```python
from build123d import *

# Parameters (mm, degrees)
ESQUISSE1_W             = 20
ESQUISSE1_H             = 20
BOSS_EXTRU_1_DEPTH      = 4
ESQUISSE4_W             = 20
ESQUISSE4_H             = 20
ESQUISSE4_W_2           = 12
ESQUISSE4_H_2           = 12
BOSS_EXTRU_2_DEPTH      = 16
ENL_V_MAT_EXTRU_2_DEPTH = 25
ENL_V_MAT_EXTRU_3_DEPTH = 25
CHANFREIN1_SIZE         = 2


with BuildPart() as part:
    # Esquisse1 → Boss.-Extru.1 (new body)
    with BuildSketch(Plane(origin=(0, 0, 0), x_dir=(1, 0, 0), z_dir=(0, 1, 0))):
        Rectangle(ESQUISSE1_W, ESQUISSE1_H)
    extrude(amount=BOSS_EXTRU_1_DEPTH)

    # Esquisse4 → Boss.-Extru.2 (add)
    with BuildSketch(Plane(origin=(0, 4, 0), x_dir=(1, 0, 0), z_dir=(0, 1, 0))):
        Rectangle(ESQUISSE4_W, ESQUISSE4_H)
        Rectangle(ESQUISSE4_W_2, ESQUISSE4_H_2, mode=Mode.SUBTRACT)
    extrude(amount=BOSS_EXTRU_2_DEPTH)

    # Esquisse5 → Enlèv. mat.-Extru.2 (cut)
    with BuildSketch(Plane.XY.offset(10)):
        Polygon((0, 14.786741301), (-5.685006524, 5.991367039), (5.739672743, 5.991367039), align=None)
    extrude(amount=-ENL_V_MAT_EXTRU_2_DEPTH, mode=Mode.SUBTRACT)

    # Esquisse6 → Enlèv. mat.-Extru.3 (cut)
    with BuildSketch(Plane(origin=(10, 0, 0), x_dir=(0, 0, -1), z_dir=(1, 0, 0))):
        Polygon((-0.002312493, 4.739245448), (5.825004197, 13.754790289), (-5.885663837, 13.754790289), align=None)
    extrude(amount=-ENL_V_MAT_EXTRU_3_DEPTH, mode=Mode.SUBTRACT)

    # Chanfrein1
    chanfrein1_edges = [part.edges().sort_by_distance(p)[0] for p in [
        (10, 10, -10),
        (10, 10, 10),
        (-10, 10, 10),
        (-10, 10, -10),
    ]]
    chamfer(chanfrein1_edges, length=CHANFREIN1_SIZE)


solid = part.part
```
Source: CAD feature listing. Evaluate the final solid. Frame: model axes, mm. A direction names the side the tool comes from. Coordinates: 2 decimals unless noted, no trailing zeros. Loops run counter-clockwise (first coordinate to the right, second up) from the corner with the lowest first, then second, coordinate; pieces in that order, holes last. Notation, with made-up numbers: M 24.5,28.5 L 53.5,28.5 A30 cw 53.5,66.5 Z; hole C -31,0.25 d2. An arc over 180 degrees is marked long. Use CSV: the item, a comma, the result in double quotes.
(1) Cut plane C-C on z = 4.5. Return loops of the section in (x, y).
Answers follow:
outline,"M -10,0 L 10,0 L 10,11.63 L 6,11.63 L 6,4 L -6,4 L -6,11.63 L -10,11.63 Z; M -10,13.75 L -6,13.75 L -6,20 L -10,20 Z; M 6,13.75 L 10,13.75 L 10,20 L 6,20 Z"
(2) Draft query along Y for faces 1 (the face through (0, 20, 7)), 2 (the face through (8.03, 9.18, -2.87)), 3 (the face through (-10, 10, 4)). Return one class per face: pulls with the +Y half, pulls with the -Y half, needs draft (parallel to the pull), parting line crosses it, or undercut.
Answers follow:
face 1,"pulls with the +Y half"
face 2,"undercut"
face 3,"needs draft"
(3) Cut plane D-D on y = 5.5. Return loops of the section in (x, z), and give its area (3 significant figures).
Answers follow:
outline,"M -10,-8 L -8,-10 L 8,-10 L 10,-8 L 10,-0.49 L 6,-0.49 L 6,-6 L -6,-6 L -6,-0.49 L -10,-0.49 Z; M -10,0.5 L -6,0.5 L -6,6 L 6,6 L 6,0.5 L 10,0.5 L 10,8 L 8,10 L -8,10 L -10,8 Z"
area,"240 mm²"
(4) Contact query for flat-ended pins moving along their axis: pin 1 (6 mm diameter, centred on x = 2, z = 1.5, fed in from +Y); pin 2 (2 mm diameter, centred on y = 8, z = -0.5, fed in from -X). Output: stop coordinate, or through.
Answers follow:
pin 1,"y = 4"
pin 2,"through"
(5) Reachability of faces 4 (the face through (-2.803, 10.451, 8.028)), 5 (the face through (-1, 14, 6)), 6 (the face through (8, 13.755, 0)) from +Z, -Z, +X, -X, +Y, -Y: full face, straight path, thin tool, end or side. Return the list, or none.
Answers follow:
face 4,"+Z, -Z"
face 5,"+Y"
face 6,"+X, -X"
(6) Cut plane A-A on x = 7.5. Return loops of the section in (y, z) (3 decimals).
Answers follow:
outline,"M 0,-10 L 20,-10 L 20,10 L 0,10 Z; hole M 4.739,0.002 L 13.755,-5.825 L 13.755,5.886 Z"
(7) Cut plane B-B on y = 16.25. Return loops of the section in (x, z), and give its area (3 significant figures).
Answers follow:
outline,"M -10,-8 L -8,-10 L 8,-10 L 10,-8 L 10,8 L 8,10 L -8,10 L -10,8 Z; hole M -6,-6 L 6,-6 L 6,6 L -6,6 Z"
area,"248 mm²"
(8) Line query: line 1 (X direction, y = 9.25, z = 5.25); line 2 (Y direction, x = -2.25, z = 3). Output: solid intervals per line, ascending. Write a range as [from, to].
Answers follow:
line 1,"[-10, -6], [6, 10]"
line 2,"[0, 4]"
